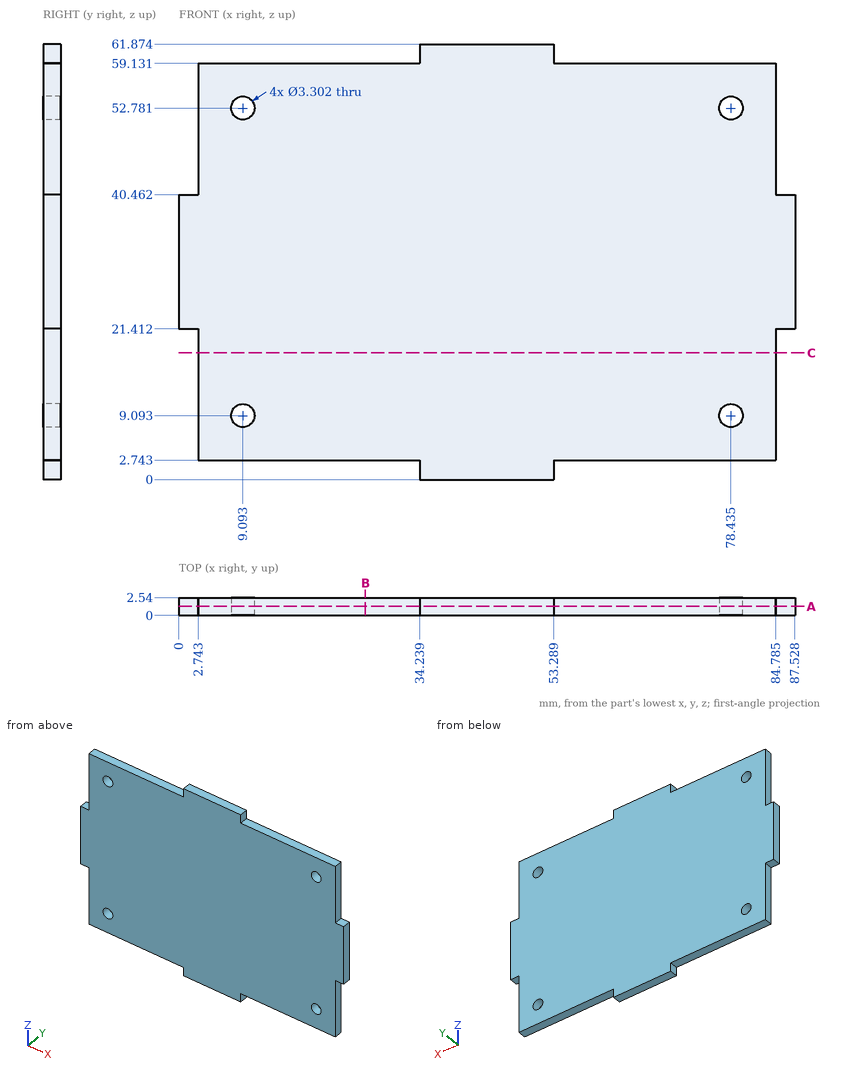
Can you work these out from the drawing? Everything is in mm from the part's minimum corner. Round coordinates to 2 decimals unless told otherwise and drop trailing zeros. Loops run counter-clockwise (first coordinate to the right, second up) from the corner with the lowest first, then second, coordinate; pieces in that order, holes last.
1. If we section it at B-B on x = 26.5: Write out the boundary of the cut face in (y, z), plus the area to 3 significant figures.
Answer list:
outline: (0, 2.74) - (2.54, 2.74) - (2.54, 59.13) - (0, 59.13) - close
area: 143 mm2
2. If I drill on line 1 along X through (y, z) = (0.2, 9) (1 decimal); line 2 along X through (y, z) = (1.85, 8) (1 decimal); line 3 along Z through (x, y) = (79, 1.65) (1 decimal), over which ranges is the centre line in solid material (lowest first)?
Answer list:
line 1: x = 2.7 to 7.4, 10.7 to 76.8, 80.1 to 84.8
line 2: x = 2.7 to 7.9, 10.3 to 77.2, 79.7 to 84.8
line 3: z = 2.7 to 7.5, 10.6 to 51.2, 54.3 to 59.1
3. If we section it at A-A on y = 1.3: Write out the boundary of the cut face in (x, z) (1 decimal), plus the area to 3 significant figures.
Answer list:
outline: (0, 21.4) - (2.7, 21.4) - (2.7, 2.7) - (34.2, 2.7) - (34.2, 0) - (53.3, 0) - (53.3, 2.7) - (84.8, 2.7) - (84.8, 21.4) - (87.5, 21.4) - (87.5, 40.5) - (84.8, 40.5) - (84.8, 59.1) - (53.3, 59.1) - (53.3, 61.9) - (34.2, 61.9) - (34.2, 59.1) - (2.7, 59.1) - (2.7, 40.5) - (0, 40.5) - close; hole circle Ø3.3 at (9.1, 9.1); hole circle Ø3.3 at (9.1, 52.8); hole circle Ø3.3 at (78.4, 9.1); hole circle Ø3.3 at (78.4, 52.8)
area: 4,800 mm2
4. If we section it at C-C on z = 18: Write out the boundary of the cut face in (x, y) (1 decimal).
Answer list:
outline: (2.7, 0) - (84.8, 0) - (84.8, 2.5) - (2.7, 2.5) - close
5. For P1, Ø1.3, axis at y = 0.5, z = 60, coming from the +X side; P2, Ø1.3, axis at y = 1, z = 45.5, coming from the -X side; P3, Ø4.5, axis at x = 9.09, z = 9.09, coming from the +Y side; P4, Ø1.3, axis at y = 1, z = 12.5, coming from the +X side (1 decimal), each with a flat end and sliding along its axis, tell me the tip position at first contact or that it passes through.
Answer list:
P1: stops at x = 53.29
P2: stops at x = 2.74
P3: stops at y = 2.54
P4: stops at x = 84.8
